Build history of the part. All positions in model axes, mm. Face numbers are marked on the shaded views. A direction names the side the tool comes from. Coordinates: 2 decimals unless noted, no trailing zeros. Write each loop counter-clockwise with the first axis right and the second up, starting at its lowest first coordinate (ties: lowest second). Pieces come first, ordered by that corner, then holes.
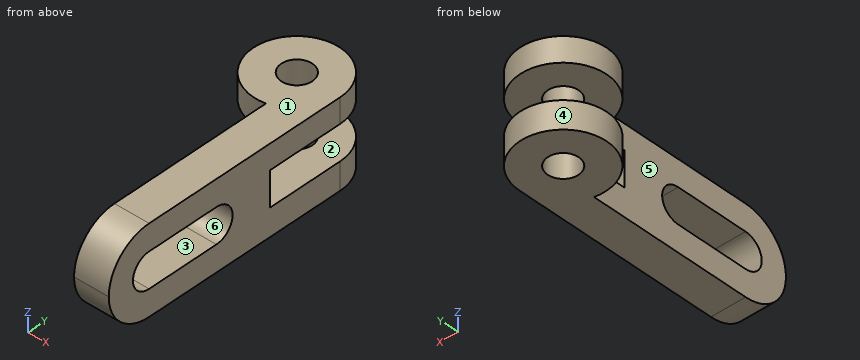
```python
from build123d import *

# Parameters (mm, degrees)
F0_R     = 5.343381
F1_DEPTH = 15
F3_W     = 41
F3_H     = 12
F4_DEPTH = 62.101


with BuildPart() as f1:
    # F0 (on Top) → F1 (new body, symmetric)
    with BuildSketch(Plane.XY):
        with BuildLine():
            Line((15, -86), (15, 0))
            ThreePointArc((15, 0), (-11.61895, 9.486833), (3, -14.696938))
            Line((3, -14.696938), (3, -86))
            Line((3, -86), (15, -86))
        make_face()
        Circle(F0_R, mode=Mode.SUBTRACT)
    extrude(amount=F1_DEPTH, both=True)

    # F3 (on offset) → F4 (cut, through all)
    with BuildSketch(Plane.YZ.offset(-47.1)):
        with Locations((-5.5, 0.449385)):
            Rectangle(F3_W, F3_H)
        with BuildLine():
            Line((-71, -6), (-46, -6))
            ThreePointArc((-46, -6), (-40, 0), (-46, 6))
            Line((-46, 6), (-71, 6))
            ThreePointArc((-71, 6), (-77, 0), (-71, -6))
        make_face()
        with BuildLine():
            Line((-86, -15), (-71, -15))
            ThreePointArc((-71, -15), (-81.606602, -10.606602), (-86, 0))
            Line((-86, 0), (-86, -15))
        make_face()
        with BuildLine():
            Line((-86, 15), (-86, 0))
            ThreePointArc((-86, 0), (-81.606602, 10.606602), (-71, 15))
            Line((-71, 15), (-86, 15))
        make_face()
    extrude(amount=F4_DEPTH, mode=Mode.SUBTRACT)


solid = f1.part
```
1. Saw through at A-A on x = 0. List the corners of the cut face in (y, z).
Computed values:
outline: (-15, -15) - (-5.34, -15) - (-5.34, -5.55) - (-15, -5.55) - close; (-15, 6.45) - (-5.34, 6.45) - (-5.34, 15) - (-15, 15) - close; (5.34, -15) - (15, -15) - (15, -5.55) - (5.34, -5.55) - close; (5.34, 6.45) - (15, 6.45) - (15, 15) - (5.34, 15) - close
2. Mould opens along Y. For the marked faces 4, 5 and 6 say: +Y half, -Y half, draft (parallel to the pull), parting line (faces both ways), or undercut.
Computed values:
face 4: parting line
face 5: draft
face 6: undercut
3. Saw through at D-D on x = 12.5. List the corners of the cut face in (y, z), plus the area to 3 significant figures.
Computed values:
outline: (-86, 0) arc R15 ccw to (-71, -15) - (8.29, -15) - (8.29, -5.55) - (-26, -5.55) - (-26, 6.45) - (8.29, 6.45) - (8.29, 15) - (-71, 15) arc R15 ccw to start; hole (-71, -6) - (-46, -6) arc R6 ccw to (-46, 6) - (-71, 6) arc R6 ccw to start
area: 1,910 mm2
4. Probe line 1 along X through (y, z) = (0, -8); line 2 along Z through (x, y) = (-11.5, 1.5). List the from-to ranges inside material, lowest first.
Computed values:
line 1: x = -15 to -5.34, 5.34 to 15
line 2: z = -15 to -5.55, 6.45 to 15
5. Flat gauge pins, fed straight in: pin 1 (5 mm diameter, centred on x = -0.5, y = -29, fed in from -Z); pin 2 (8 mm diameter, centred on x = -11, z = 4, fed in from -Y); pin 3 (5 mm diameter, centred on x = -8.5, z = 12, fed in from +Y); pin 4 (2 mm diameter, centred on y = -75.5, z = -11, fed in from -X). Where does each tip first touch, or does it go through?
Computed values:
pin 1: passes through
pin 2: stops at y = -12.79
pin 3: stops at y = 13.75
pin 4: stops at x = 3
6. Saw through at C-C on z = -3. List the corners of the cut face in (x, y), plus the area to 3 significant figures.
Computed values:
outline: (3, -85.7) - (15, -85.7) - (15, -76.2) - (3, -76.2) - close; (3, -40.8) - (15, -40.8) - (15, -26) - (3, -26) - close
area: 292 mm2
7. 3-axis set-ups, long thin cutter, end or side, ignore diameter. For the marked faces 1, 2 and 3: which of +Z, -Z, +X, -X, +Y, -Y reach the whole face in a straight line?
Computed values:
face 1: +Z, +X, -X, +Y, -Y
face 2: +X, -X, +Y
face 3: +X, -X
8. Saw through at B-B on y = -17.5. List the corners of the cut face in (x, z).
Computed values:
outline: (3, -15) - (15, -15) - (15, -5.55) - (3, -5.55) - close; (3, 6.45) - (15, 6.45) - (15, 15) - (3, 15) - close
